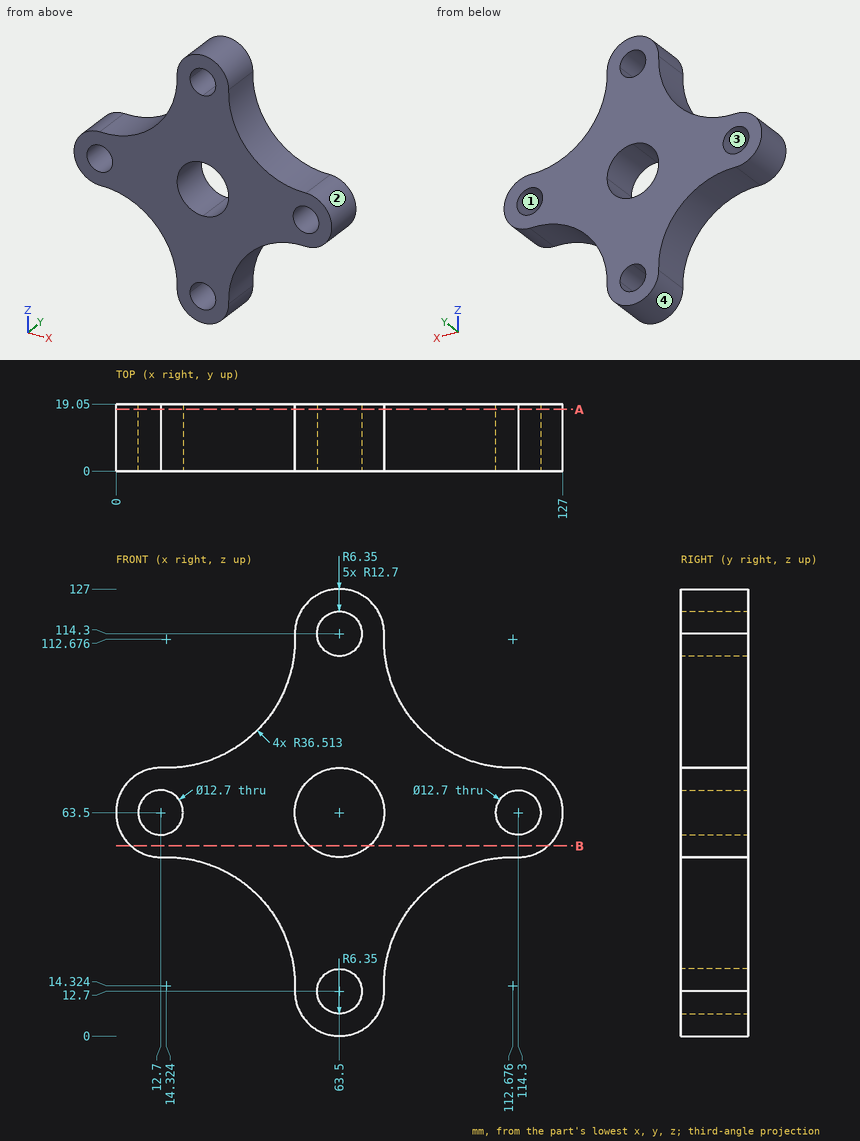
Can you work these out from the drawing? Everything is in mm from the part's minimum corner. Round coordinates to 2 decimals unless told otherwise and drop trailing zeros. Order: outer loops, then holes, each group sorted by start corner. A loop starts at its lowest first (then second) coordinate and runs counter-clockwise, first axis right, second up. Notation, with made-up numbers: (27, 57.5) -> (79, 57.5) arc R35 cw to (79, 96.5) -> close; hole circle Ø9 at (2, 40). An arc over 180 degrees is marked (long way). Return JSON: item names as keys, results as strings. Group by question number.
1. I need wall thicknesses on line 1 (Z direction, x = 114.3, y = 4); line 2 (Z direction, x = 66.5, y = 5.25) (1 decimal); line 3 (X direction, y = 15.25, z = 110.5) (1 decimal). Which ranges of each line are inside material? Lowest first, please. Write a range as [from, to].
2. If we section it at A-A, the plane y = 17.5: Count the separate pieces of the cut face and the enclosed holes in it, then the cut area to 3 significant figures.
3. If we section it at B-B, the plane z = 54: Write out the boundary of the cut face in (x, y), then the cut area to 3 significant figures.
4. Will these pins go through, and if not, where does the flat tip stop? pin 1 (4 mm diameter, centred on x = 19.5, y = 8.5, fed in from +Z); pin 2 (8 mm diameter, centred on x = 96.5, y = 4.5, fed in from -Z) (1 decimal); pin 3 (2 mm diameter, centred on y = 5, z = 36, fed in from +X); pin 4 (7.5 mm diameter, centred on x = 12.7, z = 63.5, fed in from +Y).
5. We'd pull the mould along X, two halves only. Please class the marked faces 1, 2, 3 and 4: released by +X, released by -X, zero draft, split by the parting line, or undercut.
Output values:
{
 "1": {"line 1": "[50.8, 57.15], [69.85, 76.2]", "line 2": "[0.4, 7.1], [18.3, 51.2], [75.8, 108.7], [119.9, 126.6]", "line 3": "[50.8, 58.4], [68.6, 76.2]"},
 "2": {"separate pieces": "1", "enclosed holes": "5", "area": "5,650 mm²"},
 "3": {"outline": "(4.27, 0) -> (55.07, 0) -> (55.07, 19.05) -> (4.27, 19.05) -> close; (71.93, 0) -> (122.73, 0) -> (122.73, 19.05) -> (71.93, 19.05) -> close", "area": "1,940 mm²"},
 "4": {"pin 1": "z = 76.88", "pin 2": "z = 44.8", "pin 3": "x = 84.06", "pin 4": "through"},
 "5": {"face 1": "undercut", "face 2": "released by +X", "face 3": "undercut", "face 4": "split by the parting line"}
}
